Source: CAD feature listing. Evaluate the final solid. Frame: model axes, mm. A direction names the side the tool comes from. Coordinates: 2 decimals unless noted, no trailing zeros. Order: outer loops, then holes, each group sorted by start corner. A loop starts at its lowest first (then second) coordinate and runs counter-clockwise, first axis right, second up. Notation, with made-up numbers: (-28.5, 83.25) - (-7.5, 83.25) arc R7 ccw to (-7.5, 96.25) - close; hole circle Ø11 at (82, 18). An arc over 180 degrees is marked (long way). One line per question, with ' | ' between items. Start each with the question number.
(1) Draft query along X for faces 4 (the flat face through (17, 100, 37.592)), 5 (the flat face through (150.673, 46, 25)), 6 (the flat face through (136.703, 97, 42)), 7 (the flat face through (132, 99.441, 42)). Return one class per face: +X half, -X half, draft (parallel to the pull), parting line (faces both ways), or undercut.
(2) Contact query for flat-ended pins moving along their axis: P1, Ø1.7, axis at y = 96, z = 41, coming from the +X side; P2, Ø7, axis at x = 132.5, y = 98, coming from the +Z side; P3, Ø6, axis at y = 97, z = 43.5, coming from the -X side. Output: stop coordinate, or through.
(3) Section B-B (z = 16.5). Return the cut outline in (x, y).
(4) Access query for faces 1 (the flat face through (17, 100, 45.53)), 2 (the flat face through (13.97, 97, 42)), 3 (the flat face through (134, 100, 37.592)). Directions: +Z, -Z, +X, -X, +Y, -Y. A direction counts if a zero-diameter tool reaches every point of the face in a straight line with its end or side. Return the directions, or none.
(5) Section C-C (x = 37). Return the cut outline in (y, z).
(6) Line query: line 1 along Y through (x, z) = (71, 44). Output: solid intervals per line, ascending.
(7) Section A-A (x = 20.5). Return the cut outline in (y, z), then the cut area to 3 significant figures.
from build123d import *

# Parameters (mm, degrees)
SKETCH2_W      = 150.6728
SKETCH2_H      = 93.853
EXTRUDE1_DEPTH = 50.292
SKETCH3_W      = 0.889
SKETCH3_H      = 7.9375
EXTRUDE2_DEPTH = 6.477
SKETCH5_W      = 11.049
SKETCH5_H      = 7.9375
EXTRUDE3_DEPTH = 0.889


with BuildPart() as part:
    # Sketch2 → Extrude1 (new body)
    with BuildSketch(Plane.XY):
        with Locations((75.3364, 46.9265)):
            Rectangle(SKETCH2_W, SKETCH2_H)
    extrude(amount=EXTRUDE1_DEPTH)

    # Sketch3 → Extrude2 (add)
    with BuildSketch(Plane(origin=(0, 93.853, 0), x_dir=(-1, 0, 0), z_dir=(0, 1, 0))):
        with Locations((-13.5255, 41.56075)):
            Rectangle(SKETCH3_W, SKETCH3_H)
        with Locations((-137.1473, 41.56075)):
            Rectangle(SKETCH3_W, SKETCH3_H)
    extrude(amount=EXTRUDE2_DEPTH)

    # Sketch5 → Extrude3 (add)
    with BuildSketch(Plane(origin=(0, 100.33, 0), x_dir=(-1, 0, 0), z_dir=(0, 1, 0))):
        with Locations((-18.6055, 41.56075)):
            Rectangle(SKETCH5_W, SKETCH5_H)
        with Locations((-132.0673, 41.56075)):
            Rectangle(SKETCH5_W, SKETCH5_H)
    extrude(amount=-EXTRUDE3_DEPTH)


solid = part.part
Response values:
1) face 4: draft | face 5: +X half | face 6: undercut | face 7: undercut
2) P1: stops at x = 137.59 | P2: stops at z = 45.53 | P3: stops at x = 13.08
3) outline: (0, 0) - (150.67, 0) - (150.67, 93.85) - (0, 93.85) - close
4) face 1: +Z, +X, -X, +Y | face 2: +Z, -Z | face 3: -Z, +X, -X, +Y
5) outline: (0, 0) - (93.85, 0) - (93.85, 50.29) - (0, 50.29) - close
6) line 1: y = 0 to 93.85
7) outline: (0, 0) - (93.85, 0) - (93.85, 50.29) - (0, 50.29) - close; (99.44, 37.59) - (100.33, 37.59) - (100.33, 45.53) - (99.44, 45.53) - close | area: 4,730 mm²
